Part print with two shaded views. Sizes in mm from the minimum x, y, z corner. Round coordinates to 2 decimals unless told otherwise and drop trailing zeros. Loops run counter-clockwise (first coordinate to the right, second up) from the corner with the lowest first, then second, coordinate; pieces in that order, holes last.
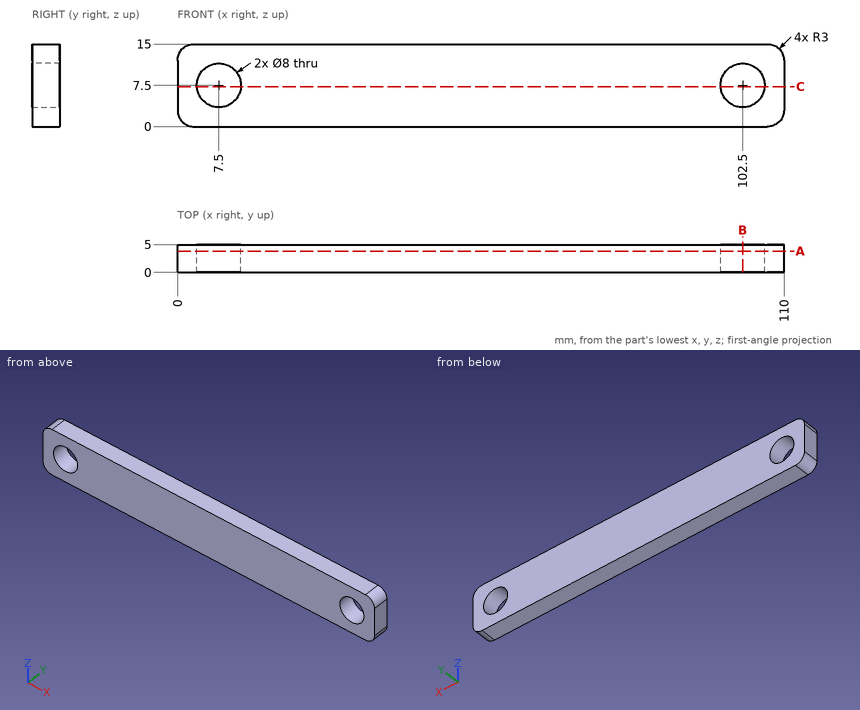
Item 1: Cut at A-A (y = 3.85). List the corners of the cut face in (x, z), plus the area to 3 significant figures.
Verdict:
outline: (0, 3) arc R3 ccw to (3, 0) - (107, 0) arc R3 ccw to (110, 3) - (110, 12) arc R3 ccw to (107, 15) - (3, 15) arc R3 ccw to (0, 12) - close; hole circle Ø8 at (7.5, 7.5); hole circle Ø8 at (102.5, 7.5)
area: 1,540 mm2
Item 2: Cut at B-B (x = 102.5). List the corners of the cut face in (y, z).
Verdict:
outline: (0, 0) - (5, 0) - (5, 3.5) - (0, 3.5) - close; (0, 11.5) - (5, 11.5) - (5, 15) - (0, 15) - close
Item 3: Cut at C-C (z = 7.25). List the corners of the cut face in (x, y).
Verdict:
outline: (0, 0) - (3.51, 0) - (3.51, 5) - (0, 5) - close; (11.49, 0) - (98.51, 0) - (98.51, 5) - (11.49, 5) - close; (106.49, 0) - (110, 0) - (110, 5) - (106.49, 5) - close
Item 4: Wall check: L1, parallel to X at y = 2.9, z = 7.5; L2, parallel to X at y = 0.7, z = 4.25; L3, parallel to Z at x = 11, y = 4.7. Give the ranges that are in metal, low to high.
Verdict:
L1: x = 0 to 3.5, 11.5 to 98.5, 106.5 to 110
L2: x = 0 to 5.17, 9.83 to 100.17, 104.83 to 110
L3: z = 0 to 5.56, 9.44 to 15
